Geometry check sheet. Reference: the model listing, model coordinates, mm. Face numbers are marked on the shaded views. Coordinates: 2 decimals unless noted, no trailing zeros. Loops run counter-clockwise (first coordinate to the right, second up) from the corner with the lowest first, then second, coordinate; pieces in that order, holes last.
from build123d import *

# Parameters (mm, degrees)
SKETCH1_R           = 50
SKETCH1_R_2         = 30
BOSS_EXTRUDE1_DEPTH = 20
SKETCH2_R           = 60
BOSS_EXTRUDE4_DEPTH = 50
BOSS_EXTRUDE4_TAPER = 40
SKETCH5_R           = 60
SKETCH5_R_2         = 55
BOSS_EXTRUDE5_DEPTH = 20
SKETCH6_R           = 1
CUT_EXTRUDE1_DEPTH  = 51.0000001


with BuildPart() as part:
    # Sketch1 → Boss-Extrude1 (new body)
    with BuildSketch(Plane(origin=(0, 0, 0), x_dir=(0, 0, -1), z_dir=(1, 0, 0))):
        Circle(SKETCH1_R)
        Circle(SKETCH1_R_2, mode=Mode.SUBTRACT)
    extrude(amount=BOSS_EXTRUDE1_DEPTH)

    # Sketch2 → Boss-Extrude4 (add)
    with BuildSketch(Plane(origin=(20, 0, 0), x_dir=(0, 0, -1), z_dir=(1, 0, 0))):
        Circle(SKETCH2_R)
    extrude(amount=BOSS_EXTRUDE4_DEPTH, taper=BOSS_EXTRUDE4_TAPER)

    # Sketch5 → Boss-Extrude5 (add)
    with BuildSketch(Plane.ZY.offset(-20)):
        Circle(SKETCH5_R)
        Circle(SKETCH5_R_2, mode=Mode.SUBTRACT)
    extrude(amount=BOSS_EXTRUDE5_DEPTH)

    # Sketch6 → Cut-Extrude1 (cut, through all)
    with BuildSketch(Plane.ZY.offset(-20)):
        Circle(SKETCH6_R)
    extrude(amount=-CUT_EXTRUDE1_DEPTH, mode=Mode.SUBTRACT)


solid = part.part
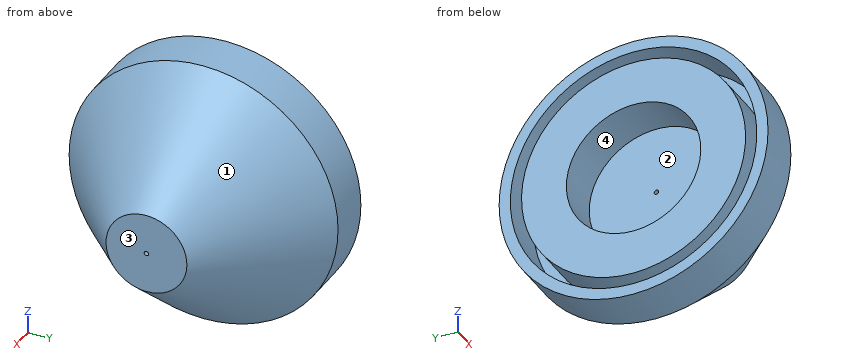
(1) Scan lines: L1, parallel to Y at x = 11.25, z = 0; L2, parallel to Z at x = 13.5, y = -19; L3, parallel to Y at x = 10, z = 16. Record each from-to range of solid material in increasing order.
Findings:
L1: y = -60 to -55, -50 to -30, 30 to 50, 55 to 60
L2: z = -56.91 to -51.61, -46.25 to -23.22, 23.22 to 46.25, 51.61 to 56.91
L3: y = -57.83 to -52.62, -47.37 to -25.38, 25.38 to 47.37, 52.62 to 57.83
(2) Sectioned sample at B-B on x = 54. Record the cut outline in (y, z).
Findings:
outline: circle Ø62.94 at (0, 0); hole circle Ø2 at (0, 0)
(3) Sectioned sample at A-A on x = 30. Record the cut outline in (y, z), and give its area (3 significant figures).
Findings:
outline: circle Ø103.22 at (0, 0); hole circle Ø2 at (0, 0)
area: 8,360 mm2
(4) Gauge pin test, flat ends, axial feed: pin 1 Ø8 at (y, z) = (-13, 31.5) entering from +X; pin 2 Ø4 at (y, z) = (-18, -42.5) entering from +X; pin 3 Ø10 at (x, y) = (8, -34) entering from -Z. Record the tip position at first contact, or that the pin passes through.
Findings:
pin 1: stops at x = 55.66
pin 2: stops at x = 38.88
pin 3: stops at z = -52.53
(5) Draft check along Y on the marked faces 1, 2, 3 and 4. Enter one of: +Y half, -Y half, draft (parallel to the pull), parting line (faces both ways), or undercut.
Findings:
face 1: parting line
face 2: undercut
face 3: draft
face 4: undercut
